Work out the finished part from the listing and answer in its coordinate system (mm). Face numbers are marked on the shaded views. A direction names the side the tool comes from. Coordinates: 2 decimals unless noted, no trailing zeros. Write each loop counter-clockwise with the first axis right and the second up, starting at its lowest first coordinate (ties: lowest second). Pieces come first, ordered by that corner, then holes. Notation, with made-up numbers: M 34.25,32 L 79.25,32 A32 cw 79.25,58 Z; hole C -31.5,56.5 d7. An arc over 180 degrees is marked long. Use CSV: the item, a comma, the result in double quotes.
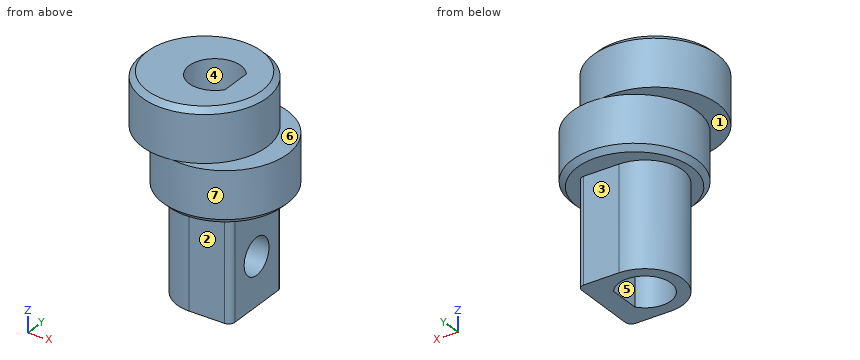
from build123d import *

# Parameters (mm, degrees)
SKETCH10_R                     = 6
BOSS_EXTRUDE4_DEPTH            = 5
BOSS_EXTRUDE5_DEPTH            = 10
SKETCH16_R                     = 6
BOSS_EXTRUDE6_DEPTH            = 5
CUT_EXTRUDE2_DEPTH             = 23.360679775
F_3_5_3_5_DIAMETER_HOLE0_D     = 3.5
F_3_5_3_5_DIAMETER_HOLE0_DEPTH = 4
F_3_5_3_5_DIAMETER_HOLE0_TIP   = 1.051506083
CHAMFER2_SIZE                  = 0.5


with BuildPart() as part:
    # Sketch10 → Boss-Extrude4 (new body)
    with BuildSketch(Plane.XY.offset(0.4)):
        Circle(SKETCH10_R)
    extrude(amount=BOSS_EXTRUDE4_DEPTH)

    # Sketch11 → Boss-Extrude5 (add)
    with BuildSketch(Plane(origin=(0, 0, 0.4), x_dir=(-1, 0, 0), z_dir=(0, 0, -1))):
        with BuildLine():
            Line((-3, -3.05), (-3, 3.05))
            ThreePointArc((-3, 3.05), (-2.824264069, 3.474264069), (-2.4, 3.65))
            Line((-2.4, 3.65), (1, 3.65))
            ThreePointArc((1, 3.65), (4.65, 0), (1, -3.65))
            Line((1, -3.65), (-2.4, -3.65))
            ThreePointArc((-2.4, -3.65), (-2.824264069, -3.474264069), (-3, -3.05))
        make_face()
    extrude(amount=BOSS_EXTRUDE5_DEPTH)

    # Sketch16 → Boss-Extrude6 (add)
    with BuildSketch(Plane(origin=(0, 0, 5.4), x_dir=(-1, 0, 0), z_dir=(0, 0, -1))):
        with Locations((2, 0)):
            Circle(SKETCH16_R)
    extrude(amount=-BOSS_EXTRUDE6_DEPTH)

    # Sketch17 → Cut-Extrude2 (cut, through all)
    with BuildSketch(Plane.XY.offset(-9.6)):
        with BuildLine():
            Line((1, -1.5), (1, 1.5))
            ThreePointArc((1, 1.5), (-3.5, 0), (1, -1.5))
        make_face()
    extrude(amount=CUT_EXTRUDE2_DEPTH, mode=Mode.SUBTRACT)

    # Ø3.5 (3.5) Diameter Hole0
    with Locations(Plane(origin=(3, 0, 0), x_dir=(0, 0, -1), z_dir=(1, 0, 0))):
        with Locations((5, 0)):
            Hole(F_3_5_3_5_DIAMETER_HOLE0_D / 2, depth=F_3_5_3_5_DIAMETER_HOLE0_DEPTH)
            with Locations((0, 0, -(F_3_5_3_5_DIAMETER_HOLE0_DEPTH + F_3_5_3_5_DIAMETER_HOLE0_TIP / 2))):  # 118° drill point
                Cone(0, F_3_5_3_5_DIAMETER_HOLE0_D / 2, F_3_5_3_5_DIAMETER_HOLE0_TIP, mode=Mode.SUBTRACT)

    # Chamfer2
    chamfer2_edges = [part.edges().sort_by_distance(p)[0] for p in [
        (-6, 0, 0.4),
        (4, 0, 10.4),
    ]]
    chamfer(chamfer2_edges, length=CHAMFER2_SIZE)


solid = part.part
Item 1: A tool of negligible diameter and unlimited length cuts with its end or side. For the marked faces 1, 2 and 3, from which of +Z, -Z, +X, -X, +Y, -Y can it reach the whole face along a straight path? Write none if from no direction.
Answer:
face 1,"-Z, -X"
face 2,"-Z, +X, -X, -Y"
face 3,"-Z, +X, -X, +Y"
Item 2: The part is cut by section A-A (z = -2.75). Write down the section's boundary in (x, y), then the cut area to 3 significant figures.
Answer:
outline,"M -1,-3.65 L 2.4,-3.65 A0.6 ccw 3,-3.05 L 3,3.05 A0.6 ccw 2.4,3.65 L -1,3.65 A3.65 ccw Z; hole M 1,-1.5 L 1,1.5 A2.5 ccw long Z"
area,"31.4 mm2"
Item 3: The part is cut by section B-B (z = -5). Write down the section's boundary in (x, y), then the cut area to 3 significant figures.
Answer:
outline,"M -1,-3.65 L 2.4,-3.65 A0.6 ccw 3,-3.05 L 3,-1.75 L 0.79,-1.75 A2.5 cw long 0.79,1.75 L 3,1.75 L 3,3.05 A0.6 ccw 2.4,3.65 L -1,3.65 A3.65 ccw Z"
area,"24.3 mm2"
Item 4: Consider probe 1 along Y at (x, z) = (2.15, -5); probe 2 along Z at (x, y) = (1.4, 0); probe 3 along Y at (x, z) = (0.25, -8). Determine where each line is inside the solid, lowest interval first.
Answer:
probe 1,"y = -3.65 to -1.75, 1.75 to 3.65"
probe 2,"z = -9.6 to -6.75, -3.25 to 10.4"
probe 3,"y = -3.65 to -2.17, 2.17 to 3.65"
Item 5: The part is cut by section C-C (z = 8.5). Write down the section's boundary in (x, y), then the cut area to 3 significant figures.
Answer:
outline,"C -2,0 d12; hole M 1,-1.5 L 1,1.5 A2.5 ccw long Z"
area,"94.5 mm2"
Item 6: For a pull along X with two mould halves and no side action, classify the marked faces 4, 5, 6 and 7 as released by +X, released by -X, zero draft, split by the parting line, or undercut.
Answer:
face 4,"undercut"
face 5,"undercut"
face 6,"zero draft"
face 7,"split by the parting line"
Item 7: Given pin 1 (2.5 mm diameter, centred on y = 0.5, z = -8, fed in from -X); pin 2 (1.7 mm diameter, centred on x = 0.5, z = -3.5, fed in from -Y); pin 3 (1 mm diameter, centred on y = 4, z = 5.5, fed in from +X), each flat-ended and moving along its own axis, determine where each tip first touches the part or whether it passes through.
Answer:
pin 1,"stops at x = -4.65"
pin 2,"stops at y = -3.65"
pin 3,"stops at x = 4.87"
